from build123d import *

# Parameters (mm, degrees)
F0_W     = 101.6
F0_H     = 101.6
F1_DEPTH = 139.7
F2_SIZE  = 10.16
F3_R     = 22.86
F4_DEPTH = 38.1
F5_R     = 12.7
F6_DEPTH = 12.7


with BuildPart() as f1:
    # F0 (on Top) → F1 (new body)
    with BuildSketch(Plane.XY):
        Rectangle(F0_W, F0_H)
    extrude(amount=F1_DEPTH)

    # F2
    f2_edges = [f1.edges().sort_by_distance(p)[0] for p in [
        (0, -50.8, 139.7),
        (-50.8, 0, 139.7),
        (50.8, 0, 139.7),
        (0, 50.8, 139.7),
        (-50.8, 50.8, 69.85),
        (50.8, 50.8, 69.85),
        (50.8, -50.8, 69.85),
        (-50.8, -50.8, 69.85),
    ]]
    chamfer(f2_edges, length=F2_SIZE)

    # F3 (on face) → F4 (cut)
    with BuildSketch(Plane.XY.offset(139.7)):
        Circle(F3_R)
    extrude(amount=-F4_DEPTH, mode=Mode.SUBTRACT)

    # F5 (on face) → F6 (cut)
    with BuildSketch(Plane(origin=(0, 0, 0), x_dir=(1, 0, 0), z_dir=(0, 0, -1))):
        Circle(F5_R)
    extrude(amount=-F6_DEPTH, mode=Mode.SUBTRACT)


solid = f1.part
Geometry: final body of the model. Coordinates: model frame, mm. A direction names the side the tool comes from. Give positions to 0.01 mm unless a question says otherwise; leave off trailing zeros. Write each loop counter-clockwise with the first axis right and the second up, starting at its lowest first coordinate (ties: lowest second). Pieces come first, ordered by that corner, then holes.
(1) Cut plane A-A, the plane z = 108. Return loops of the section in (x, y), then the cut area to 3 significant figures.
(2) Cut plane C-C, the plane z = 51. Return loops of the section in (x, y).
(3) Cut plane B-B, the plane x = 0. Return loops of the section in (y, z).
(4) Access query for faces 1 (the flat face through (45.65, -0.57, 134.69)), 2 (the cylindrical face through (21.804, 6.867, 120.917)), 3 (the flat face through (0, 0, 12.7)). Directions: +Z, -Z, +X, -X, +Y, -Y. A direction counts if a zero-diameter tool reaches every point of the face in a straight line with its end or side. Return the directions, or none.
(5) Ray query, line 1 (Y direction, x = 0, z = 129); line 2 (Y direction, x = 0, z = 7.25). Return the intervals inside material, ascending.
(6) First-contact query: P1, Ø2, axis at x = 5.5, y = -2.5, coming from the +Z side. Flat tip, straight axial feed; report the tip coordinate or a pass-through.
(7) Mould query, pull axis Y, two halves, no side actions, for faces 4 (the flat face through (-45.65, -45.79, 63.86)), 5 (the flat face through (0, 0, 101.6)), 6 (the flat face through (-50.8, -1, 64)). Classes: released by +Y, released by -Y, zero draft, split by the parting line, or undercut.
Values follow:
1. outline: (-50.8, -40.64) - (-40.64, -50.8) - (40.64, -50.8) - (50.8, -40.64) - (50.8, 40.64) - (40.64, 50.8) - (-40.64, 50.8) - (-50.8, 40.64) - close; hole circle Ø45.72 at (0, 0)
1. area: 8,470 mm2
2. outline: (-50.8, -40.64) - (-40.64, -50.8) - (40.64, -50.8) - (50.8, -40.64) - (50.8, 40.64) - (40.64, 50.8) - (-40.64, 50.8) - (-50.8, 40.64) - close
3. outline: (-50.8, 0) - (-12.7, 0) - (-12.7, 12.7) - (12.7, 12.7) - (12.7, 0) - (50.8, 0) - (50.8, 129.54) - (40.64, 139.7) - (22.86, 139.7) - (22.86, 101.6) - (-22.86, 101.6) - (-22.86, 139.7) - (-40.64, 139.7) - (-50.8, 129.54) - close
4. face 1: +Z, +X, +Y, -Y
4. face 2: +Z
4. face 3: -Z
5. line 1: y = -50.8 to -22.86, 22.86 to 50.8
5. line 2: y = -50.8 to -12.7, 12.7 to 50.8
6. P1: stops at z = 101.6
7. face 4: released by -Y
7. face 5: undercut
7. face 6: zero draft
